For this review, take the finished solid that the model builds, in its own axes (mm). A direction names the side the tool comes from. Give positions to 0.01 mm unless a question says otherwise; leave off trailing zeros. Order: outer loops, then holes, each group sorted by start corner. A loop starts at its lowest first (then second) coordinate and runs counter-clockwise, first axis right, second up. Notation, with made-up numbers: (45, 70.5) - (95, 70.5) arc R7 cw to (95, 74.5) - close; hole circle Ø2 at (86.25, 37.25). An arc over 180 degrees is marked (long way). One line per item, written item: value.
```python
from build123d import *

# Parameters (mm, degrees)
F0_R     = 15
F1_DEPTH = 30
F2_DEPTH = 10
F3_R     = 5
F4_DEPTH = 20.8588644763


with BuildPart() as f1:
    # F0 (on Right) → F1 (new body, symmetric)
    with BuildSketch(Plane.YZ):
        with BuildLine():
            ThreePointArc((95, 30), (90, 15), (95, 0))
            ThreePointArc((95, 0), (134.6047593344, -0.5130078141), (125, 37.9128784748))
            Line((125, 37.9128784748), (125, 50))
            Line((125, 50), (105, 50))
            Line((105, 50), (105, 37.9128784748))
            ThreePointArc((105, 37.9128784748), (99.4869921859, 34.6047593344), (95, 30))
        make_face()
        with Locations((115, 15)):
            Circle(F0_R, mode=Mode.SUBTRACT)
    extrude(amount=F1_DEPTH, both=True)

    # F0 (on Right) → F2 (join, symmetric)
    with BuildSketch(Plane.YZ):
        with BuildLine():
            ThreePointArc((15, 30), (0, 15), (15, 0))
            Line((15, 0), (65, 0))
            ThreePointArc((65, 0), (75, 10), (85, 0))
            Line((85, 0), (95, 0))
            ThreePointArc((95, 0), (90, 15), (95, 30))
            Line((95, 30), (85, 30))
            ThreePointArc((85, 30), (75, 20), (65, 30))
            Line((65, 30), (15, 30))
        make_face()
        with BuildLine():
            ThreePointArc((15, 7), (7, 15), (15, 23))
            Line((15, 23), (35, 23))
            ThreePointArc((35, 23), (43, 15), (35, 7))
            Line((35, 7), (15, 7))
        make_face(mode=Mode.SUBTRACT)
    extrude(amount=F2_DEPTH, both=True)

    # F3 (on face) → F4 (cut, through all)
    with BuildSketch(Plane.XY.offset(50)):
        with Locations((15, 115)):
            Circle(F3_R)
        with Locations((-15, 115)):
            Circle(F3_R)
    extrude(amount=-F4_DEPTH, mode=Mode.SUBTRACT)


solid = f1.part
```
(1) Take a section at D-D (x = -3). Write out the cut boundary in (y, z).
Answers below:
outline: (15, 0) - (65, 0) arc R10 cw to (85, 0) - (95, 0) arc R25 ccw (long way) to (125, 37.91) - (125, 50) - (105, 50) - (105, 37.91) arc R25 ccw to (95, 30) - (85, 30) arc R10 cw to (65, 30) - (15, 30) arc R15 ccw to start; hole (15, 7) - (35, 7) arc R8 ccw to (35, 23) - (15, 23) arc R8 ccw to start; hole circle Ø30 at (115, 15)
(2) For P1, Ø1.5, axis at x = -19.5, z = 9, coming from the -Y side; P2, Ø4, axis at x = 1, y = 23.5, coming from the -Z side; P3, Ø8, axis at x = -21.5, z = 39, coming from the -Y side, all flat-tipped, find the tip position at first contact; note any pin that passes through.
Answers below:
P1: stops at y = 90.56
P2: stops at z = 0
P3: stops at y = 100
(3) Take a section at C-C (z = 44.5). Write out the cut boundary in (x, y), then the cut area to 3 significant figures.
Answers below:
outline: (-30, 105) - (30, 105) - (30, 125) - (-30, 125) - close; hole circle Ø10 at (-15, 115); hole circle Ø10 at (15, 115)
area: 1,040 mm^2
(4) Machinability: for faces 1 (the face through (19.77, 116.5, 39.72)), 2 (the face through (0, 105, 44)), 3 (the face through (0, 75, 20)), 4 (the face through (0, 43, 15)), 5 (the face through (0, 40, 0)), which of the approach directions +Z, -Z, +X, -X, +Y, -Y give a long, thin tool a straight path to every point of the face, cutting with its end or side? Answer none if there is none.
Answers below:
face 1: +Z
face 2: +Z, +X, -X, -Y
face 3: +Z, +X, -X
face 4: +X, -X
face 5: -Z, +X, -X, -Y
(5) Take a section at B-B (y = 127). Write out the cut boundary in (x, z), then the cut area to 3 significant figures.
Answers below:
outline: (-30, -6.93) - (30, -6.93) - (30, 6) - (-30, 6) - close; (-30, 24) - (30, 24) - (30, 36.93) - (-30, 36.93) - close
area: 1,550 mm^2
(6) Take a section at A-A (x = -15). Write out the cut boundary in (y, z).
Answers below:
outline: (105, 37.91) arc R25 ccw (long way) to (125, 37.91) - (125, 50) - (120, 50) - (120, 29.14) arc R15 cw (long way) to (110, 29.14) - (110, 50) - (105, 50) - close
(7) Wall thickness on line 1 (X direction, y = 115, z = 36); line 2 (Y direction, x = -15, z = 45); line 3 (Z direction, x = 9, y = 115): over which ranges is each line inside the solid? List them lowest first. Write a range as from..to.
Answers below:
line 1: x = -30..-20, -10..10, 20..30
line 2: y = 105..110, 120..125
line 3: z = -10..0, 30..50
(8) Draft analysis for pull direction Y (two halves, no side actions). For faces 6 (the face through (10, 47, 15)), 7 (the face through (0, 0, 15)), 8 (the face through (0, 25, 23)), 9 (the face through (-16.08, 110.12, 39.72)), state which applies: pulls with the +Y half, pulls with the -Y half, needs draft (parallel to the pull), parting line crosses it, or undercut.
Answers below:
face 6: needs draft
face 7: pulls with the -Y half
face 8: undercut
face 9: undercut
